from build123d import *

# Parameters (mm, degrees)
RAIL_W                    = 3.2
RAIL_H                    = 1.5
RAIL_W_2                  = 1.5
RAIL_H_2                  = 3
RAIL_W_3                  = 10.292519685
BOSS_EXTRUDE1_DEPTH       = 350
BOSS_EXTRUDE2_OUTLINE_W   = 350
BOSS_EXTRUDE2_OUTLINE_H   = 4.5
BOSS_EXTRUDE2_DEPTH       = 1.5
BOSS_EXTRUDE2_2_OUTLINE_W = 350
BOSS_EXTRUDE2_2_OUTLINE_H = 4.5
BOSS_EXTRUDE2_2_DEPTH     = 1.5
FILLET1_R                 = 4
FILLET2_R                 = 4
BOSS_EXTRUDE3_DEPTH       = 3
FILLET3_R                 = 1
FILLET4_R                 = 1
LPATTERN1_COUNT           = 2
LPATTERN1_PITCH           = 353


# Read off the part's stored shape, not the designer's step: Boss-Extrude2
with BuildPart() as part:
    # rail → Boss-Extrude1 (new body)
    with BuildSketch(Plane.XY):
        with Locations((0, -24.462398)):
            Rectangle(RAIL_W, RAIL_H)
        Polygon((1.6, -23.712398), (1.6, -25.212398), (1.6, -26.712398), (3.1, -26.712398), (3.1, -23.712398), align=None)
        with Locations((4.442519685, -25.21)):
            Rectangle(RAIL_W_2, RAIL_H_2)
        with Locations((5.942519685, -24.46)):
            Rectangle(RAIL_W_2, RAIL_H)
        with Locations((5.942519685, -131.96)):
            Rectangle(RAIL_W_2, RAIL_H)
        with Locations((4.442519685, -131.21)):
            Rectangle(RAIL_W_2, RAIL_H_2)
        Polygon((1.6, -129.710002609), (1.6, -131.210002609), (1.6, -132.710002609), (3.1, -132.710002609), (3.1, -129.710002609), align=None)
        with Locations((0, -131.960002609)):
            Rectangle(RAIL_W, RAIL_H)
        with Locations((1.546259843, -22.96)):
            Rectangle(RAIL_W_3, RAIL_H)
        with Locations((1.546259843, -133.46)):
            Rectangle(RAIL_W_3, RAIL_H)
    extrude(amount=-BOSS_EXTRUDE1_DEPTH)

    # Boss-Extrude2 outline → Boss-Extrude2 (add)
    with BuildSketch(Plane(origin=(6.692519685, 0, 0), x_dir=(0, 0, -1), z_dir=(1, 0, 0))):
        with Locations((175, -24.46)):
            Rectangle(BOSS_EXTRUDE2_OUTLINE_W, BOSS_EXTRUDE2_OUTLINE_H)
    extrude(amount=BOSS_EXTRUDE2_DEPTH)

    # Fillet1
    fillet1_edges = [part.edges().sort_by_distance(p)[0] for p in [
        (8.192519685, -22.21, -175),
    ]]
    fillet(fillet1_edges, radius=FILLET1_R)



with BuildPart() as body_2:
    # Boss-Extrude2 2 outline → Boss-Extrude2 2 (new body)
    with BuildSketch(Plane(origin=(6.692519685, 0, 0), x_dir=(0, 0, -1), z_dir=(1, 0, 0))):
        with Locations((175, -131.96)):
            Rectangle(BOSS_EXTRUDE2_2_OUTLINE_W, BOSS_EXTRUDE2_2_OUTLINE_H)
    extrude(amount=BOSS_EXTRUDE2_2_DEPTH)

    # Fillet2
    # the kernel refuses this fillet: 4 mm, written as the material it takes off along each edge
    with BuildSketch(Plane(origin=(8.192519685, -134.21, 7.806247498), x_dir=(-1, 0, 0), z_dir=(0, 0, -1))) as fillet2_piece_1:
        with BuildLine():
            CenterArc((4, 3.122498999), FILLET2_R, 180, 51.317812547)
            Line((0, 3.122498999), (-0.08, 3.122498999))
            Line((-0.08, 3.122498999), (-0.08, 0))
            Line((-0.08, 0), (0, -0.08))
            ThreePointArc((0, -0.08), (0.75, -0.08), (1.45, -0.06244998))
            Line((1.45, -0.06244998), (1.5, 0))
        make_face()
    extrude(amount=365.612494996, mode=Mode.SUBTRACT)


with BuildPart() as part_1:
    add(part.part)

    add(body_2.part)  # Boss-Extrude3 merges body 2
    # side → Boss-Extrude3 (add)
    with BuildSketch(Plane.XY):
        with BuildLine():
            Line((8.192519685, -26.71), (8.192519685, -129.71))
            Line((8.192519685, -129.71), (8.192519685, -131.087501001))
            ThreePointArc((8.192519685, -131.087501001), (7.798070961, -132.819551808), (6.692519685, -134.21))
            Line((6.692519685, -134.21), (-3.6, -134.21))
            ThreePointArc((-3.6, -134.21), (-5.909675728, -133.059247145), (-7.060428583, -130.749571417))
            Line((-7.060428583, -130.749571417), (-14.282896215, -79.148969011))
            Line((-14.282896215, -79.148969011), (-20.976742465, -31.325078818))
            ThreePointArc((-20.976742465, -31.325078818), (-19.494827467, -25.608174313), (-14.404493379, -22.613584515))
            Line((-14.404493379, -22.613584515), (-3.6, -22.21))
            Line((-3.6, -22.21), (4.192519685, -22.21))
            ThreePointArc((4.192519685, -22.21), (7.04796816, -23.699601355), (8.192519685, -26.71))
        make_face()
    boss_extrude3 = extrude(amount=BOSS_EXTRUDE3_DEPTH)

    # Fillet3
    fillet3_edges = [part_1.edges().sort_by_distance(p)[0] for p in [
        (8.192519685, -129.71, -175),
    ]]
    fillet(fillet3_edges, radius=FILLET3_R)

    # Fillet4
    # the kernel refuses this fillet: 1 mm, written as the material it takes off along each edge
    with BuildSketch(Plane(origin=(8.192519685, -26.71, 0), x_dir=(-0.047899365984683646, 0.9988521666083853, 0), z_dir=(0, 0, -1))) as fillet4_piece_1:
        with BuildLine():
            CenterArc((1.048761395, -0.992864746), FILLET4_R, 83.151413818, 99.594068227)
            Line((0.049909229, -1.040764112), (-0.049975988, -1.045554048))
            Line((-0.049975988, -1.045554048), (-0.099885217, -0.004789937))
            Line((-0.099885217, -0.004789937), (-0.004789937, 0.099885217))
            ThreePointArc((-0.004789937, 0.099885217), (0.494636147, 0.1238349), (1.179931939, 0.099286475))
            Line((1.179931939, 0.099286475), (1.168007344, 0))
        make_face()
    extrude(amount=352.920018361, mode=Mode.SUBTRACT)

    # LPattern1: Boss-Extrude3 ×2
    with Locations(*[(0, 0, -i * LPATTERN1_PITCH) for i in range(1, LPATTERN1_COUNT)]):
        add(boss_extrude3)


solid = part_1.part
Input: part model. Units: mm. Frame: model coordinates. A direction names the side the tool comes from. Round coordinates to 2 decimals unless told otherwise and drop trailing zeros. Order: outer loops, then holes, each group sorted by start corner. A loop starts at its lowest first (then second) coordinate and runs counter-clockwise, first axis right, second up. Notation, with made-up numbers: (1, 77.25) - (47, 77.25) arc R20 ccw to (47, 86.25) - close; hole circle Ø11 at (60.5, 36.5). An arc over 180 degrees is marked (long way). Answer as a JSON object with one key per item and string values. Group by question number.
(1) Reachability of faces 1 (the face through (-2, -23.71, -173)), 2 (the face through (0, -22.21, -177)) from +Z, -Z, +X, -X, +Y, -Y: full face, straight path, thin tool, end or side. Return the list, or none.
(2) Cut plane B-B (z = -143). Count the separate pieces of the cut face and the enclosed holes in it, then the cut area to 3 significant figures.
(3) Draft query along Y for faces 3 (the face through (2, -134.21, -177)), 4 (the face through (-3, -65, -353)), 5 (the face through (-3, -65, -350)). Return one class per face: released by +Y, released by -Y, zero draft, split by the parting line, or undercut.
(4) Pin query (flat end, axial travel): P1, Ø0.8, axis at y = -25.5, z = -217.5, coming from the +X side; P2, Ø0.8, axis at y = -26, z = -94, coming from the -X side; P3, Ø0.8, axis at y = -23, z = -225.5, coming from the -X side. Return the tip coordinate at first contact, or that it passes through.
(5) Cut plane C-C (y = -62.5). Return loops of the section in (x, z), then the cut area to 3 significant figures.
(6) Material intervals for probe 1 along Y at (x, z) = (-3.25, -29); probe 2 along Z at (x, y) = (-4.75, -69.5), sorted ascending. Write a range as from..to.
(7) Cut plane A-A (y = -125.5). Return loops of the section in (x, z), then the cut area to 3 significant figures.
Here are the results:
{
 "1": {"face 1": "none", "face 2": "+Z, -Z, +X, -X, +Y"},
 "2": {"separate pieces": "3", "enclosed holes": "0", "area": "71.2 mm^2"},
 "3": {"face 3": "released by -Y", "face 4": "zero draft", "face 5": "undercut"},
 "4": {"P1": "stops at x = 8.15", "P2": "stops at x = 1.6", "P3": "stops at x = -3.6"},
 "5": {"outline": "(-16.61, -353) - (8.19, -353) - (8.19, -350) - (-16.61, -350) - close; (-16.61, 0) - (8.19, 0) - (8.19, 3) - (-16.61, 3) - close", "area": "149 mm^2"},
 "6": {"probe 1": "y = -134.21..-132.71, -23.71..-22.21", "probe 2": "z = -353..-350, 0..3"},
 "7": {"outline": "(-7.8, -353) - (8.19, -353) - (8.19, -350) - (-7.8, -350) - close; (-7.8, 0) - (8.19, 0) - (8.19, 3) - (-7.8, 3) - close", "area": "95.9 mm^2"}
}
